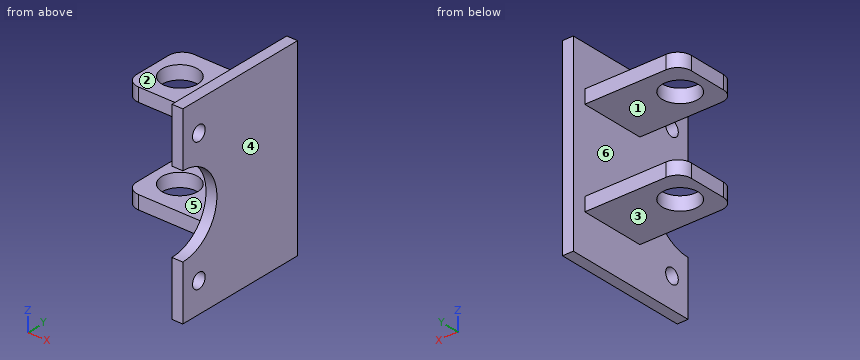
```python
from build123d import *

# Parameters (mm, degrees)
SKETCH003_W   = 24
SKETCH003_H   = 5
PAD002_DEPTH  = 35
SKETCH004_R   = 6.6
HOLE001_DEPTH = 5.001
FILLET002_R   = 5
FILLET003_R   = 5
SKETCH002_W   = 24
SKETCH002_H   = 5
PAD001_DEPTH  = 35
SKETCH005_R   = 6.6
HOLE002_DEPTH = 5.001
FILLET_R      = 5
FILLET001_R   = 5
SKETCH_W      = 50
SKETCH_H      = 70
PAD_DEPTH     = 4
SKETCH001_R   = 2.75
HOLE_DEPTH    = 4.001
SKETCH006_R   = 14.85
HOLE003_DEPTH = 4.001


with BuildPart() as body002:
    # Sketch003 (on Face1 of CopyHole001) → Pad002 (new body)
    with BuildSketch(Plane(origin=(0, 0, 0), x_dir=(0, 1, 0), z_dir=(-1, 0, 0))):
        with Locations((63, -52.5)):
            Rectangle(SKETCH003_W, SKETCH003_H)
    extrude(amount=PAD002_DEPTH)

    # Sketch004 (on Face3 of Pad002) → Hole001 (cut, through all)
    with BuildSketch(Plane(origin=(0, 0, 55), x_dir=(0, -1, 0), z_dir=(0, 0, 1))):
        with Locations((-63, -25)):
            Circle(SKETCH004_R)
    extrude(amount=-HOLE001_DEPTH, mode=Mode.SUBTRACT)

    # Fillet002
    fillet002_edges = [body002.edges().sort_by_distance(p)[0] for p in [
        (-35, 75, 52.5),
    ]]
    fillet(fillet002_edges, radius=FILLET002_R)

    # Fillet003
    fillet003_edges = [body002.edges().sort_by_distance(p)[0] for p in [
        (-35, 51, 52.5),
    ]]
    fillet(fillet003_edges, radius=FILLET003_R)


with BuildPart() as body001:
    # Sketch002 (on Face1 of CopyHole) → Pad001 (new body)
    with BuildSketch(Plane(origin=(0, 0, 0), x_dir=(0, 1, 0), z_dir=(-1, 0, 0))):
        with Locations((63, -17.5)):
            Rectangle(SKETCH002_W, SKETCH002_H)
    extrude(amount=PAD001_DEPTH)

    # Sketch005 (on Face3 of Pad001) → Hole002 (cut, through all)
    with BuildSketch(Plane(origin=(0, 0, 20), x_dir=(0, -1, 0), z_dir=(0, 0, 1))):
        with Locations((-63, -25)):
            Circle(SKETCH005_R)
    extrude(amount=-HOLE002_DEPTH, mode=Mode.SUBTRACT)

    # Fillet
    fillet_edges = [body001.edges().sort_by_distance(p)[0] for p in [
        (-35, 75, 17.5),
    ]]
    fillet(fillet_edges, radius=FILLET_R)

    # Fillet001
    fillet001_edges = [body001.edges().sort_by_distance(p)[0] for p in [
        (-35, 51, 17.5),
    ]]
    fillet(fillet001_edges, radius=FILLET001_R)


with BuildPart() as body:
    # Sketch → Pad (new body)
    with BuildSketch(Plane.YZ):
        with Locations((55, 35)):
            Rectangle(SKETCH_W, SKETCH_H)
    extrude(amount=PAD_DEPTH)

    # Sketch001 (on Face5 of Pad) → Hole (cut, through all)
    with BuildSketch(Plane(origin=(0, 0, 0), x_dir=(0, 1, 0), z_dir=(-1, 0, 0))):
        with Locations((37, -11)):
            Circle(SKETCH001_R)
        with Locations((37, -59)):
            Circle(SKETCH001_R)
    extrude(amount=-HOLE_DEPTH, mode=Mode.SUBTRACT)

    # Sketch006 (on Face4 of Hole) → Hole003 (cut, through all)
    with BuildSketch(Plane(origin=(0, 0, 0), x_dir=(0, 1, 0), z_dir=(-1, 0, 0))):
        with Locations((30, -35)):
            Circle(SKETCH006_R)
    extrude(amount=-HOLE003_DEPTH, mode=Mode.SUBTRACT)

    # Boolean: union Body002, Body001
    add(body002.part)
    add(body001.part)


solid = body.part
```
Verification items for the finished model (mm, model axes). Face numbers are marked on the shaded views. A direction names the side the tool comes from. Give positions to 0.01 mm unless a question says otherwise; leave off trailing zeros. Write each loop counter-clockwise with the first axis right and the second up, starting at its lowest first coordinate (ties: lowest second). Pieces come first, ordered by that corner, then holes. Notation, with made-up numbers: (5.25, 60) - (20.25, 60) arc R36 cw to (20.25, 96) - close; hole circle Ø3 at (68.25, 77). An arc over 180 degrees is marked (long way). Put each result on its own line as item: value.
Q1. Set-up check for the marked faces 1 and 2: record each of +Z, -Z, +X, -X, +Y, -Y from which the full face is reachable in a straight line by a thin tool's end or side.
Result:
face 1: -X, +Y, -Y
face 2: +Z, -X, +Y, -Y
Q2. Section check C-C on y = 63. Record the cut outline in (x, z).
Result:
outline: (-35, 15) - (-31.6, 15) - (-31.6, 20) - (-35, 20) - close; (-35, 50) - (-31.6, 50) - (-31.6, 55) - (-35, 55) - close; (-18.4, 15) - (0, 15) - (0, 0) - (4, 0) - (4, 70) - (0, 70) - (0, 55) - (-18.4, 55) - (-18.4, 50) - (0, 50) - (0, 20) - (-18.4, 20) - close
Q3. Scan lines: probe 1 along Z at (x, y) = (-31, 66.5); probe 2 along X at (y, z) = (63, 16); probe 3 along Z at (x, y) = (1.25, 37). Record each from-to range of solid material in increasing order. Write a range as from..to.
Result:
probe 1: 15..20, 50..55
probe 2: -35..-31.6, -18.4..4
probe 3: 0..8.25, 13.75..21.9, 48.1..56.25, 61.75..70
Q4. Depth check by flat-ended pin: P1, Ø12, axis at x = -11, y = 63.5, coming from the -Z side; P2, Ø2, axis at y = 73.5, z = 14.5, coming from the -X side; P3, Ø5.5, axis at x = -16.5, z = 53.5, coming from the +Y side. Enter the tip coordinate at first touch or a pass-through.
Result:
P1: z = 15
P2: x = -34.25
P3: y = 75
Q5. Mould release check, pull along Z, two halves, no side actions. Record for the marked faces 3, 4, 5 and 6: released by +Z, released by -Z, zero draft, split by the parting line, or undercut.
Result:
face 3: released by -Z
face 4: zero draft
face 5: undercut
face 6: undercut
Q6. Section check D-D on x = -10.5. Record the cut outline in (y, z).
Result:
outline: (51, 15) - (75, 15) - (75, 20) - (51, 20) - close; (51, 50) - (75, 50) - (75, 55) - (51, 55) - close
Q7. Section check B-B on z = 52.5. Record the cut outline in (x, y), and give its area (3 significant figures).
Result:
outline: (-35, 56) arc R5 ccw to (-30, 51) - (0, 51) - (0, 30) - (4, 30) - (4, 80) - (0, 80) - (0, 75) - (-30, 75) arc R5 ccw to (-35, 70) - close; hole circle Ø13.2 at (-25, 63)
area: 892 mm2
Q8. Section check A-A on x = -25. Record the cut outline in (y, z).
Result:
outline: (51, 15) - (56.4, 15) - (56.4, 20) - (51, 20) - close; (51, 50) - (56.4, 50) - (56.4, 55) - (51, 55) - close; (69.6, 15) - (75, 15) - (75, 20) - (69.6, 20) - close; (69.6, 50) - (75, 50) - (75, 55) - (69.6, 55) - close
